from build123d import *

# Parameters (mm, degrees)
CROQUIS1_W              = 5
CROQUIS1_H              = 5
SALIENTE_EXTRUIR1_DEPTH = 3


with BuildPart() as part:
    # Croquis1 → Saliente-Extruir1 (new body)
    with BuildSketch(Plane.XY):
        with Locations((-10.453849245, 5.502257497)):
            Rectangle(CROQUIS1_W, CROQUIS1_H)
        Polygon((-7.953849245, 9.002257497), (-7.953849245, 8.002257497), (-7.953849245, 3.002257497), (-7.953849245, 2.002257497), (-5.953849245, 2.002257497), (-5.953849245, 9.002257497), align=None)
    extrude(amount=SALIENTE_EXTRUIR1_DEPTH)


solid = part.part
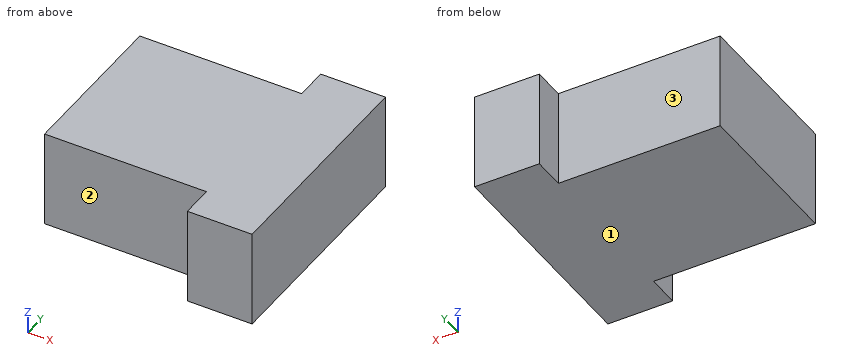
Check sheet for the modelled part. Datum: model origin and axes. Units: mm. Face numbers are marked on the shaded views. A direction names the side the tool comes from. Give positions to 0.01 mm unless a question says otherwise; leave off trailing zeros. Loops run counter-clockwise (first coordinate to the right, second up) from the corner with the lowest first, then second, coordinate; pieces in that order, holes last. Notation, with made-up numbers: M -26.75,-30.75 L -4.75,-30.75 A17 ccw -4.75,-14.75 Z; hole C 45,-27.5 d8. An arc over 180 degrees is marked long. Return JSON: item names as keys, results as strings. Group by question number.
1. Cross-section at B-B on x = -10.5. Record the boundary of the cut face in (y, z), plus the area to 3 significant figures.
2. Thickness scan on L1, parallel to X at y = 8.75, z = 2.35; L2, parallel to Y at x = -9.75, z = 2.45. Record the ranges inside material, lowest first.
3. Tool access check on the marked faces 1, 2 and 3. Record the directions out of +Z, -Z, +X, -X, +Y, -Y that give a thin tool (end or side, any length) a straight path to the whole face; none if there is none.
4. Cross-section at A-A on z = 1. Record the boundary of the cut face in (x, y), plus the area to 3 significant figures.
5. Go/stop test with flat-tipped pins: pin 1 (0.9 mm diameter, centred on x = -9.5, z = 2, fed in from +Y); pin 2 (1.5 mm diameter, centred on x = -10, z = 2, fed in from -Y); pin 3 (0.5 mm diameter, centred on y = 8.5, z = 1, fed in from -X). Record where each tip stops, or that it passes through.
Return value:
{
 "1": {"outline": "M 3,0 L 8,0 L 8,3 L 3,3 Z", "area": "15.0 mm^2"},
 "2": {"L1": "-7.95 to -5.95", "L2": "3 to 8"},
 "3": {"face 1": "-Z, +X, -X, +Y, -Y", "face 2": "+Z, -Z, -X, -Y", "face 3": "+Z, -Z, -X, +Y"},
 "4": {"outline": "M -12.95,3 L -7.95,3 L -7.95,2 L -5.95,2 L -5.95,9 L -7.95,9 L -7.95,8 L -12.95,8 Z", "area": "39.0 mm^2"},
 "5": {"pin 1": "y = 8", "pin 2": "y = 3", "pin 3": "x = -7.95"}
}
